Can you work these out from the model? Positions are in its coordinate system, mm. Face numbers are marked on the shaded views. A direction names the side the tool comes from. Give positions to 0.01 mm unless a question says otherwise; leave off trailing zeros. Order: outer loops, then holes, each group sorted by start corner. A loop starts at its lowest first (then second) coordinate and runs counter-clockwise, first axis right, second up. Notation, with made-up numbers: (-0.5, -38) - (50.5, -38) arc R5 cw to (50.5, -32) - close; hole circle Ø8 at (-4.5, -18). An arc over 180 degrees is marked (long way). Answer as CSV lines item,"result".
```python
from build123d import *

# Parameters (mm, degrees)
SKETCH_1_R          = 2
EXTRUDE_1_DEPTH     = 10
SKETCH_2_R          = 3.5
EXTRUDE_2_DEPTH     = 3.91
CUT_EXTRUDE_1_DEPTH = 2


with BuildPart() as part:
    # 草图1 → 凸台-拉伸1 (new body)
    with BuildSketch(Plane(origin=(0, 0, 0), x_dir=(1, 0, 0), z_dir=(0, 1, 0))):
        Circle(SKETCH_1_R)
    extrude(amount=EXTRUDE_1_DEPTH)

    # 草图2 → 凸台-拉伸2 (add)
    with BuildSketch(Plane(origin=(0, 10, 0), x_dir=(1, 0, 0), z_dir=(0, 1, 0))):
        Circle(SKETCH_2_R)
    extrude(amount=EXTRUDE_2_DEPTH)

    # 草图3 → 切除-拉伸1 (cut)
    with BuildSketch(Plane(origin=(0, 13.91, 0), x_dir=(1, 0, 0), z_dir=(0, 1, 0))):
        Polygon((1.669374847, -1.13864874), (1.820786158, 0.876396656), (0.151411311, 2.015045396), (-1.669374847, 1.13864874), (-1.820786158, -0.876396656), (-0.151411311, -2.015045396), align=None)
    extrude(amount=-CUT_EXTRUDE_1_DEPTH, mode=Mode.SUBTRACT)


solid = part.part
```
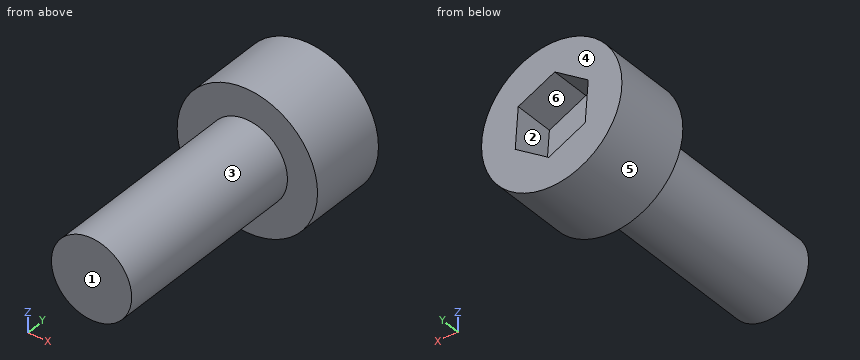
1) If we mould it in two halves opening along X, with no side actions, what happens to the marked faces 4, 5 and 6? For each: +X half, -X half, draft (parallel to the pull), parting line (faces both ways), or undercut.
Answer block:
face 4,"draft"
face 5,"parting line"
face 6,"undercut"
2) I want a section at A-A on x = 0.75. Write out the boundary of the cut face in (y, z), plus the area to 3 significant figures.
Answer block:
outline,"(0, -1.85) - (10, -1.85) - (10, -3.42) - (13.91, -3.42) - (13.91, -1.61) - (11.91, -1.61) - (11.91, 1.58) - (13.91, 1.58) - (13.91, 3.42) - (10, 3.42) - (10, 1.85) - (0, 1.85) - close"
area,"57.4 mm2"
3) I want a section at C-C on y = 5. Write out the boundary of the cut face in (x, z).
Answer block:
outline,"circle Ø4 at (0, 0)"
4) Which directions (+Z, -Z, +X, -X, +Y, -Y) give clear straight access to the entire face, cutting with the end or side of a thin tool? Please do the marked faces 1, 2 and 3.
Answer block:
face 1,"+Z, -Z, +X, -X, -Y"
face 2,"+Y"
face 3,"-Y"
5) I want a section at D-D on x = -3. Write out the boundary of the cut face in (y, z).
Answer block:
outline,"(10, -1.8) - (13.91, -1.8) - (13.91, 1.8) - (10, 1.8) - close"
6) I want a section at B-B on z = 0. Write out the boundary of the cut face in (x, y), plus the area to 3 significant figures.
Answer block:
outline,"(-3.5, 10) - (-2, 10) - (-2, 0) - (2, 0) - (2, 10) - (3.5, 10) - (3.5, 13.91) - (1.75, 13.91) - (1.75, 11.91) - (-1.75, 11.91) - (-1.75, 13.91) - (-3.5, 13.91) - close"
area,"60.4 mm2"
7) I'm going to push flat-ended pins straight in: P1, Ø1.1, axis at x = 0, z = 1, coming from the +Y side; P2, Ø3, axis at y = 3.5, z = -1, coming from the -X side; P3, Ø2, axis at x = 1, y = 4, coming from the +Z side. Where does each tip first touch, or does it pass through?
Answer block:
P1,"y = 11.91"
P2,"x = -2"
P3,"z = 2"
8) I need wall thicknesses on line 1 along Y through (x, z) = (-2.5, 2); line 2 along Y through (x, z) = (-0.25, 0.25); line 3 along Z through (x, y) = (-1.75, 6). Which ranges of each line are inside material? Lowest first, please. Write a range as [from, to].
Answer block:
line 1,"[10, 13.91]"
line 2,"[0, 11.91]"
line 3,"[-0.97, 0.97]"
